from build123d import *

# Parameters (mm, degrees)
F0_W      = 40
F0_H      = 30
F0_R      = 1.56
F1_DEPTH  = 6.25
F2_R      = 6.55
F4_W      = 5
F4_H      = 25
F5_DEPTH  = 20
F6_R      = 5
F7_R      = 1.2
F9_W      = 2.5
F9_H      = 2
F10_DEPTH = 36
F11_R     = 5
F12_DEPTH = 15.5


with BuildPart() as f1:
    # F0 (on Top) → F1 (new body)
    with BuildSketch(Plane.XY):
        Rectangle(F0_W, F0_H)
        with Locations((13.459221, -8.45)):
            Circle(F0_R, mode=Mode.SUBTRACT)
        with Locations((13.466984, 8.45)):
            Circle(F0_R, mode=Mode.SUBTRACT)
    extrude(amount=F1_DEPTH)

    # F2
    f2_edges = [f1.edges().sort_by_distance(p)[0] for p in [
        (-20, -15, 3.125),
        (-20, 15, 3.125),
        (20, -15, 3.125),
        (20, 15, 3.125),
    ]]
    fillet(f2_edges, radius=F2_R)

    # F4 (on offset) → F5 (join)
    with BuildSketch(Plane.XY.offset(5.8)):
        Rectangle(F4_W, F4_H)
    extrude(amount=F5_DEPTH)

    # F6
    f6_edges = [f1.edges().sort_by_distance(p)[0] for p in [
        (0, 12.5, 25.8),
        (0, -12.5, 25.8),
    ]]
    fillet(f6_edges, radius=F6_R)

    # F7
    f7_edges = [f1.edges().sort_by_distance(p)[0] for p in [
        (0, -12.5, 6.25),
        (0, 12.5, 6.25),
    ]]
    fillet(f7_edges, radius=F7_R)

    # F9 (on offset) → F10 (cut)
    with BuildSketch(Plane.XZ.offset(15.1)):
        with Locations((-9.976846, 1)):
            Rectangle(F9_W, F9_H)
    extrude(amount=-F10_DEPTH, mode=Mode.SUBTRACT)

    # F11 (on Right) → F12 (cut, symmetric)
    with BuildSketch(Plane.YZ):
        with Locations((0, 15.371925)):
            Circle(F11_R)
    extrude(amount=F12_DEPTH, both=True, mode=Mode.SUBTRACT)


solid = f1.part
Could you check a few things on this model? Use its own coordinates, in mm. A direction names the side the tool comes from. Give positions to 0.01 mm unless a question says otherwise; leave off trailing zeros. Order: outer loops, then holes, each group sorted by start corner. A loop starts at its lowest first (then second) coordinate and runs counter-clockwise, first axis right, second up.
1. We'd pull the mould along Y, two halves only. Please class faces 1 (the cylindrical face through (18.03, 13.13, 3.17)), 2 (the flat face through (20, 0, 3)), 3 (the cylindrical face through (0.04, -0.65, 20.33)): pulls with the +Y half, pulls with the -Y half, needs draft (parallel to the pull), parting line crosses it, or undercut.
2. Suppose I cut it at A-A (y = 0). List the corners of the cut face in (x, z) for me.
3. Will these pins go through, and if not, where does the flat tip stop? P1, Ø4, axis at x = 0.5, z = 14.5, coming from the +Y side; P2, Ø6, axis at y = 0, z = 15.37, coming from the -X side; P3, Ø1.5, axis at x = 0.5, z = 13.5, coming from the -Y side; P4, Ø6, axis at y = 6.5, z = 19, coming from the +X side.
4. I need wall thicknesses on L1, parallel to Z at x = -1.05, y = 0; L2, parallel to Z at x = 11.5, y = 11; L3, parallel to Y at x = 2, z = 10.25. Which ranges of each line are inside material? Lowest first, please.
5. Suppose I cut it at B-B (z = 19.25). List the corners of the cut face in (x, y) for me, plus the area to 3 significant figures.
6. Suppose I cut it at C-C (z = 2.75). List the corners of the cut face in (x, y) for me.
7. For faces 4 (the flat face through (0, -12.5, 14)), 5 (the cylindrical face through (-18.13, 13.03, 3.17)), 6 (the cylindrical face through (0.04, 11.07, 24.3)), 7 (the flat face through (-10, 0, 2)), 8 (the flat face through (2.5, 3, 20)), which set-ups out of +Z, -Z, +X, -X, +Y, -Y let a thin tool reach every point of the face, with its end or its side?
8. Suppose I cut it at D-D (x = 0.5). List the corners of the cut face in (y, z) for me.
Solved:
1. face 1: pulls with the +Y half
1. face 2: needs draft
1. face 3: undercut
2. outline: (-20, 0) - (-11.23, 0) - (-11.23, 2) - (-8.73, 2) - (-8.73, 0) - (20, 0) - (20, 6.25) - (2.5, 6.25) - (2.5, 10.37) - (-2.5, 10.37) - (-2.5, 6.25) - (-20, 6.25) - close; (-2.5, 20.37) - (2.5, 20.37) - (2.5, 25.8) - (-2.5, 25.8) - close
3. P1: stops at y = 12.5
3. P2: passes through
3. P3: stops at y = -12.5
3. P4: stops at x = 2.5
4. L1: z = 0 to 10.37, 20.37 to 25.8
4. L2: z = 0 to 6.25
4. L3: y = -12.5 to 12.5
5. outline: (-2.5, -12.5) - (2.5, -12.5) - (2.5, -3.16) - (-2.5, -3.16) - close; (-2.5, 3.16) - (2.5, 3.16) - (2.5, 12.5) - (-2.5, 12.5) - close
5. area: 93.4 mm2
6. outline: (-20, -8.45) arc R6.55 ccw to (-13.45, -15) - (13.45, -15) arc R6.55 ccw to (20, -8.45) - (20, 8.45) arc R6.55 ccw to (13.45, 15) - (-13.45, 15) arc R6.55 ccw to (-20, 8.45) - close; hole circle Ø3.12 at (13.46, -8.45); hole circle Ø3.12 at (13.47, 8.45)
7. face 4: +Z, +X, -X, -Y
7. face 5: +Z, -Z, -X, +Y
7. face 6: +Z, +X, -X, +Y
7. face 7: -Z, +Y, -Y
7. face 8: +Z, +X, +Y, -Y
8. outline: (-15, 0) - (15, 0) - (15, 6.25) - (13.7, 6.25) arc R1.2 cw to (12.5, 7.45) - (12.5, 20.8) arc R5 ccw to (7.5, 25.8) - (-7.5, 25.8) arc R5 ccw to (-12.5, 20.8) - (-12.5, 7.45) arc R1.2 cw to (-13.7, 6.25) - (-15, 6.25) - close; hole circle Ø10 at (0, 15.37)
